The listing builds one solid part. Answer for the finished solid, in the listing's coordinates (mm). Face numbers are marked on the shaded views. A direction names the side the tool comes from. Round coordinates to 2 decimals unless told otherwise and drop trailing zeros. Order: outer loops, then holes, each group sorted by start corner. A loop starts at its lowest first (then second) coordinate and runs counter-clockwise, first axis right, second up. Notation, with made-up numbers: (32, 45.5) - (65, 45.5) arc R22 ccw to (65, 73.5) - close; hole circle Ø10 at (-14, 17). An arc over 180 degrees is marked (long way). One line per item, written item: value. Start each with the question number.
1. Straight lines are drawn through the part: line 1 (X direction, y = -5.4, z = 5); line 2 (X direction, y = 9.5, z = 4); line 3 (X direction, y = 7.5, z = 15.75). For each, find the intervals that lie inside material, in ascending order.
2. Section A-A, the plane y = 15 is taken. Give the vertices of the cut face in (x, z), then the cut area to 3 significant figures.
3. Section D-D, the plane z = 24.4 is taken. Give the vertices of the cut face in (x, y).
4. Section C-C, the plane y = -3.75 is taken. Give the vertices of the cut face in (x, z).
5. Flat-ended cylindrical pins translate along their axes: P1, Ø1, axis at x = 29, z = 6, coming from the +Y side; P2, Ø1, axis at x = 26, z = 13.5, coming from the +Y side; P3, Ø4.5, axis at x = 36.3, z = 5, coming from the +Y side; P4, Ø3.5, axis at x = 35.5, y = 5.5, coming from the +Z side. Find the tip coordinate at first contact, or state that the pin passes through.
6. Section B-B, the plane x = 36.3 is taken. Give the vertices of the cut face in (y, z).
7. For a pull along Z with two mould halves and no side action, classify the marked faces 1, 2, 3 and 4 as released by +Z, released by -Z, zero draft, split by the parting line, or undercut.
8. A tool of negligible diameter and unlimited length cuts with its end or side. For the marked faces 5, 6 and 7, from which of +Z, -Z, +X, -X, +Y, -Y can it reach the whole face along a straight path? Write none if from no direction.
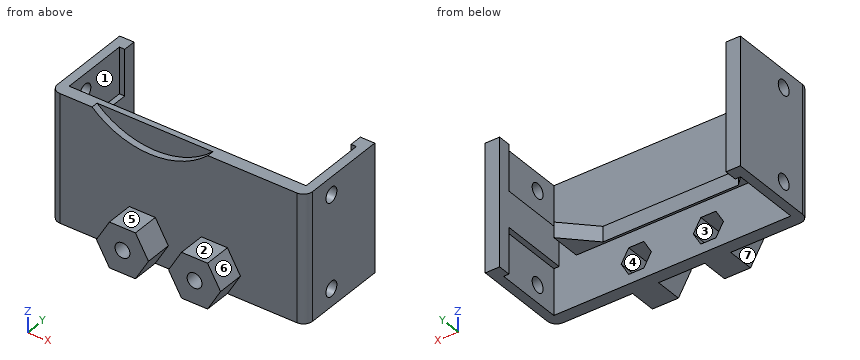
from build123d import *

# Parameters (mm, degrees)
BOSS_EXTRUDE1_DEPTH = 28.3
SKETCH2_W           = 52.58
SKETCH2_H           = 15.18
CUT_EXTRUDE1_DEPTH  = 10.2
CUT_EXTRUDE2_START  = 28.3
SKETCH2_2_W         = 52.58
SKETCH2_2_H         = 15.18
CUT_EXTRUDE2_DEPTH  = 10.2
CUT_EXTRUDE3_REACH  = 68.615
SKETCH3_R           = 1.65
BOSS_EXTRUDE2_START = 11.1
BOSS_EXTRUDE2_DEPTH = 3.4
CUT_EXTRUDE4_DEPTH  = 1.5
SKETCH6_R           = 1.65
BOSS_EXTRUDE3_DEPTH = 6
CUT_EXTRUDE5_START  = -8.82
CUT_EXTRUDE5_DEPTH  = 5.82


with BuildPart() as part:
    # Sketch1 → Boss-Extrude1 (new body)
    with BuildSketch(Plane.XY):
        with BuildLine():
            Line((0, 20.81), (3.19, 20.81))
            Line((3.19, 20.81), (3.19, 2.82))
            Line((3.19, 2.82), (53.41, 2.82))
            Line((53.41, 2.82), (53.41, 20.81))
            Line((53.41, 20.81), (56.6, 20.81))
            Line((56.6, 20.81), (56.6, 2))
            ThreePointArc((56.6, 2), (56.014213562, 0.585786438), (54.6, 0))
            Line((54.6, 0), (2, 0))
            ThreePointArc((2, 0), (0.585786438, 0.585786438), (0, 2))
            Line((0, 2), (0, 20.81))
        make_face()
    extrude(amount=BOSS_EXTRUDE1_DEPTH)

    # Sketch2 → Cut-Extrude1 (cut)
    with BuildSketch(Plane.XY):
        with Locations((28.3, 10.41)):
            Rectangle(SKETCH2_W, SKETCH2_H)
    extrude(amount=CUT_EXTRUDE1_DEPTH, mode=Mode.SUBTRACT)

    # Sketch2<2> → Cut-Extrude2 (cut)
    with BuildSketch(Plane.XY.offset(CUT_EXTRUDE2_START)):
        with Locations((28.3, 10.41)):
            Rectangle(SKETCH2_2_W, SKETCH2_2_H)
    extrude(amount=-CUT_EXTRUDE2_DEPTH, mode=Mode.SUBTRACT)

    # Cut-Extrude3: up to this face of the body (flat: up to its plane)
    cut_extrude3_end = Plane(part.part.faces().sort_by_distance((56.6, 11.405, 14.15))[0])
    # Sketch3 → Cut-Extrude3 (cut, up to the picked face)
    with BuildSketch(Plane.ZY, mode=Mode.PRIVATE) as cut_extrude3_sk1:
        with Locations((3.9, 7.71)):
            Circle(SKETCH3_R)
    cut_extrude3_tool1 = split(extrude(cut_extrude3_sk1.sketch, amount=-CUT_EXTRUDE3_REACH, mode=Mode.PRIVATE), bisect_by=cut_extrude3_end, keep=Keep.BOTH, mode=Mode.PRIVATE)
    # Sketch3 → Cut-Extrude3 (cut, up to the picked face)
    with BuildSketch(Plane.ZY, mode=Mode.PRIVATE) as cut_extrude3_sk2:
        with Locations((24.4, 7.71)):
            Circle(SKETCH3_R)
    cut_extrude3_tool2 = split(extrude(cut_extrude3_sk2.sketch, amount=-CUT_EXTRUDE3_REACH, mode=Mode.PRIVATE), bisect_by=cut_extrude3_end, keep=Keep.BOTH, mode=Mode.PRIVATE)
    add(cut_extrude3_tool1.solids().sort_by(Axis((0, 7.71, 3.9), (1, 0, 0)))[0], mode=Mode.SUBTRACT)
    add(cut_extrude3_tool2.solids().sort_by(Axis((0, 7.71, 24.4), (1, 0, 0)))[0], mode=Mode.SUBTRACT)

    # Sketch4 → Boss-Extrude2 (add)
    with BuildSketch(Plane.XY.offset(BOSS_EXTRUDE2_START)):
        Polygon((7, 9.598174593), (13.278174593, 3.32), (43.321825407, 3.32), (49.6, 9.598174593), (49.6, 2.82), (7, 2.82), align=None)
    extrude(amount=BOSS_EXTRUDE2_DEPTH)

    # Sketch5 → Cut-Extrude4 (cut)
    with BuildSketch(Plane.XZ):
        with BuildLine():
            Line((34.845232579, 28.3), (9.154767421, 28.3))
            ThreePointArc((9.154767421, 28.3), (22, 23.3), (34.845232579, 28.3))
        make_face()
    extrude(amount=-CUT_EXTRUDE4_DEPTH, mode=Mode.SUBTRACT)

    # Sketch6 → Boss-Extrude3 (add)
    # profile 1 of 2: a face of its own
    with BuildSketch(Plane.XZ):
        Polygon((26.073502692, 5), (23.186751346, 10), (17.413248654, 10), (14.526497308, 5), (17.413248654, 0), (23.186751346, 0), align=None)
        with Locations(Location((20.3, 5, 0), (0, 0, 270))):
            Circle(SKETCH6_R, mode=Mode.SUBTRACT)
    # profile 2 of 2: a face of its own
    with BuildSketch(Plane.XZ):
        Polygon((42.073502692, 5), (39.186751346, 10), (33.413248654, 10), (30.526497308, 5), (33.413248654, 0), (39.186751346, 0), align=None)
        with Locations(Location((36.3, 5, 0), (0, 0, 270))):
            Circle(SKETCH6_R, mode=Mode.SUBTRACT)
    extrude(amount=BOSS_EXTRUDE3_DEPTH)

    # Sketch8 → Cut-Extrude5 (cut)
    with BuildSketch(Plane.XZ.offset(6).offset(CUT_EXTRUDE5_START)):
        Polygon((23.648631561, 5), (21.974315781, 7.9), (18.625684219, 7.9), (16.951368439, 5), (18.625684219, 2.1), (21.974315781, 2.1), align=None)
        Polygon((39.648631561, 5), (37.974315781, 7.9), (34.625684219, 7.9), (32.951368439, 5), (34.625684219, 2.1), (37.974315781, 2.1), align=None)
    extrude(amount=CUT_EXTRUDE5_DEPTH, mode=Mode.SUBTRACT)


solid = part.part
Answer list:
1. line 1: x = 14.53 to 18.65, 21.95 to 26.07, 30.53 to 34.65, 37.95 to 42.07
1. line 2: x = 0 to 2.01, 54.59 to 56.6
1. line 3: x = 0 to 3.19, 53.41 to 56.6
2. outline: (0, 0) - (2.01, 0) - (2.01, 10.2) - (3.19, 10.2) - (3.19, 18.1) - (2.01, 18.1) - (2.01, 28.3) - (0, 28.3) - close; (53.41, 10.2) - (54.59, 10.2) - (54.59, 0) - (56.6, 0) - (56.6, 28.3) - (54.59, 28.3) - (54.59, 18.1) - (53.41, 18.1) - close
2. area: 132 mm²
3. outline: (0, 2) arc R2 ccw to (2, 0) - (15.63, 0) - (15.63, 1.5) - (28.37, 1.5) - (28.37, 0) - (54.6, 0) arc R2 ccw to (56.6, 2) - (56.6, 6.06) - (54.59, 6.06) - (54.59, 2.82) - (2.01, 2.82) - (2.01, 6.06) - (0, 6.06) - close; (0, 9.36) - (2.01, 9.36) - (2.01, 18) - (3.19, 18) - (3.19, 20.81) - (0, 20.81) - close; (53.41, 18) - (54.59, 18) - (54.59, 9.36) - (56.6, 9.36) - (56.6, 20.81) - (53.41, 20.81) - close
4. outline: (14.53, 5) - (17.41, 0) - (23.19, 0) - (26.07, 5) - (23.19, 10) - (17.41, 10) - close; (30.53, 5) - (33.41, 0) - (39.19, 0) - (42.07, 5) - (39.19, 10) - (33.41, 10) - close; hole circle Ø3.3 at (20.3, 5); hole circle Ø3.3 at (36.3, 5)
5. P1: stops at y = 2.82
5. P2: stops at y = 3.32
5. P3: stops at y = -3
5. P4: passes through
6. outline: (-6, 0) - (2.82, 0) - (2.82, 2.1) - (-3, 2.1) - (-3, 3.35) - (-6, 3.35) - close; (-6, 6.65) - (-3, 6.65) - (-3, 7.9) - (2.82, 7.9) - (2.82, 11.1) - (3.32, 11.1) - (3.32, 14.5) - (2.82, 14.5) - (2.82, 28.3) - (0, 28.3) - (0, 10) - (-6, 10) - close
7. face 1: zero draft
7. face 2: released by +Z
7. face 3: undercut
7. face 4: undercut
8. face 5: +Z, +X, -X, -Y
8. face 6: +Z, +X, -Y
8. face 7: -Z, -X, -Y
